Verification items for the finished model (mm, model axes). A direction names the side the tool comes from. Round coordinates to 2 decimals unless told otherwise and drop trailing zeros. Order: outer loops, then holes, each group sorted by start corner. A loop starts at its lowest first (then second) coordinate and runs counter-clockwise, first axis right, second up. Notation, with made-up numbers: (-18, 28) -> (19, 28) arc R21 cw to (19, 56) -> close; hole circle Ø1 at (56.5, -4). An arc over 180 degrees is marked (long way). Put each result on its own line as item: value.
```python
from build123d import *

# Parameters (mm, degrees)
PAD011_DEPTH    = 1.6
SKETCH027_R     = 1.15
POCKET013_DEPTH = 1.601
POCKET014_DEPTH = 1.601


with BuildPart() as part:
    # Sketch026 → Pad011 (new body)
    with BuildSketch(Plane.XZ):
        with BuildLine():
            Line((-12.5, 0), (12.5, 0))
            Line((12.5, 0), (12.5, 13))
            ThreePointArc((12.5, 13), (11.914214, 14.414214), (10.5, 15))
            Line((10.5, 15), (6.75, 15))
            ThreePointArc((6.75, 15), (6.396447, 14.853553), (6.25, 14.5))
            Line((6.25, 14.5), (6.25, 13.5))
            ThreePointArc((5.75, 13), (6.103553, 13.146447), (6.25, 13.5))
            Line((5.75, 13), (-5.75, 13))
            ThreePointArc((-6.25, 13.5), (-6.103553, 13.146447), (-5.75, 13))
            Line((-6.25, 13.5), (-6.25, 14.5))
            ThreePointArc((-6.25, 14.5), (-6.396447, 14.853553), (-6.75, 15))
            Line((-10.5, 15), (-6.75, 15))
            ThreePointArc((-10.5, 15), (-11.914214, 14.414214), (-12.5, 13))
            Line((-12.5, 13), (-12.5, 0))
        make_face()
    extrude(amount=PAD011_DEPTH)

    # Sketch027 → Pocket013 (cut, through all)
    with BuildSketch(Plane.XZ):
        with Locations((-10, 11)):
            Circle(SKETCH027_R)
        with Locations((10, 11)):
            Circle(SKETCH027_R)
    extrude(amount=POCKET013_DEPTH, mode=Mode.SUBTRACT)

    # Sketch028 → Pocket014 (cut, through all)
    with BuildSketch(Plane.XZ):
        with BuildLine():
            Line((7.9, 14), (7.9, 3))
            ThreePointArc((6.9, 2), (7.607107, 2.292893), (7.9, 3))
            Line((6.9, 2), (-6.9, 2))
            ThreePointArc((-7.9, 3), (-7.607107, 2.292893), (-6.9, 2))
            Line((-7.9, 3), (-7.9, 14))
            ThreePointArc((-7.9, 14), (-8.192893, 14.707107), (-8.9, 15))
            Line((-8.9, 15), (-12.5, 15))
            Line((-12.5, 15), (-12.5, 17))
            Line((-12.5, 17), (12.5, 17))
            Line((12.5, 17), (12.5, 15))
            Line((8.9, 15), (12.5, 15))
            ThreePointArc((8.9, 15), (8.192893, 14.707107), (7.9, 14))
        make_face()
    extrude(amount=POCKET014_DEPTH, mode=Mode.SUBTRACT)


solid = part.part
```
Item 1: Tool access check on faces 1 (the face through (12.5, -1, 6)), 2 (the face through (-8.185, -0.789, 14.699)). Record the directions out of +Z, -Z, +X, -X, +Y, -Y that give a thin tool (end or side, any length) a straight path to the whole face; none if there is none.
Geometry check:
face 1: +Z, -Z, +X, +Y, -Y
face 2: +Z, +Y, -Y
Item 2: Material ranges on line 1 along X through (y, z) = (-0.5, 11); line 2 along Z through (x, y) = (10, -0.7); line 3 along X through (y, z) = (-0.4, 4.75), recorded low to high.
Geometry check:
line 1: -12.5 to -11.15, -8.85 to -7.9, 7.9 to 8.85, 11.15 to 12.5
line 2: 0 to 9.85, 12.15 to 15
line 3: -12.5 to -7.9, 7.9 to 12.5
Item 3: Release check for a two-part mould opening along Z. For faces 3 (the face through (-8.938, -0.789, 10.56)), 4 (the face through (8.201, -0.789, 14.715)), 5 (the face through (-12.5, -1, 7)), 6 (the face through (0, -1, 0)) record: pulls with the +Z half, pulls with the -Z half, needs draft (parallel to the pull), parting line crosses it, or undercut.
Geometry check:
face 3: undercut
face 4: pulls with the +Z half
face 5: needs draft
face 6: pulls with the -Z half
Item 4: Depth check by flat-ended pin: pin 1 Ø3 at (x, z) = (-10, 11) entering from -Y. Enter the tip coordinate at first touch or a pass-through.
Geometry check:
pin 1: y = -1.6
Item 5: Sectioned sample at C-C, the plane x = 10. Record the boundary of the cut face in (y, z).
Geometry check:
outline: (-1.6, 0) -> (0, 0) -> (0, 9.85) -> (-1.6, 9.85) -> close; (-1.6, 12.15) -> (0, 12.15) -> (0, 15) -> (-1.6, 15) -> close
Item 6: Sectioned sample at D-D, the plane z = 3.5. Record the boundary of the cut face in (x, y), then the cut area to 3 significant figures.
Geometry check:
outline: (-12.5, -1.6) -> (-7.9, -1.6) -> (-7.9, 0) -> (-12.5, 0) -> close; (7.9, -1.6) -> (12.5, -1.6) -> (12.5, 0) -> (7.9, 0) -> close
area: 14.7 mm2
Item 7: Sectioned sample at A-A, the plane z = 11. Record the boundary of the cut face in (x, y), then the cut area to 3 significant figures.
Geometry check:
outline: (-12.5, -1.6) -> (-11.15, -1.6) -> (-11.15, 0) -> (-12.5, 0) -> close; (-8.85, -1.6) -> (-7.9, -1.6) -> (-7.9, 0) -> (-8.85, 0) -> close; (7.9, -1.6) -> (8.85, -1.6) -> (8.85, 0) -> (7.9, 0) -> close; (11.15, -1.6) -> (12.5, -1.6) -> (12.5, 0) -> (11.15, 0) -> close
area: 7.36 mm2
Item 8: Sectioned sample at B-B, the plane y = -1.05. Record the boundary of the cut face in (x, z).
Geometry check:
outline: (-12.5, 0) -> (12.5, 0) -> (12.5, 13) arc R2 ccw to (10.5, 15) -> (8.9, 15) arc R1 ccw to (7.9, 14) -> (7.9, 3) arc R1 cw to (6.9, 2) -> (-6.9, 2) arc R1 cw to (-7.9, 3) -> (-7.9, 14) arc R1 ccw to (-8.9, 15) -> (-10.5, 15) arc R2 ccw to (-12.5, 13) -> close; hole circle Ø2.3 at (-10, 11); hole circle Ø2.3 at (10, 11)
